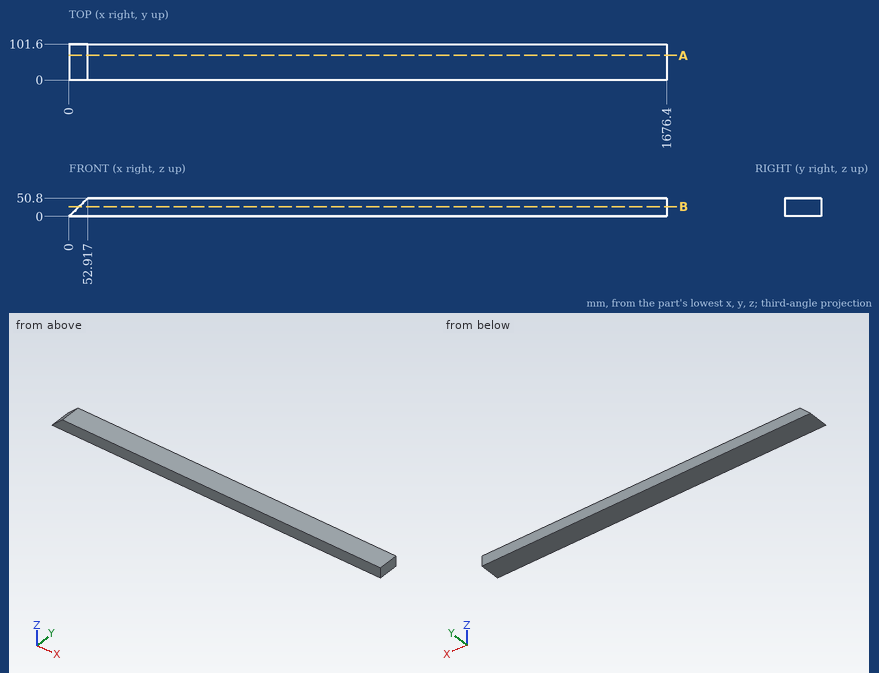
Input: dimensioned drawing with shaded views. Units: mm. Origin: part minimum x, y, z. Coordinates: 2 decimals unless noted, no trailing zeros. Write each loop counter-clockwise with the first axis right and the second up, starting at its lowest first coordinate (ties: lowest second). Pieces come first, ordered by that corner, then holes. Notation, with made-up numbers: M 28,12.25 L 36,12.25 A15 cw 36,34.25 Z; hole C 48.25,-10 d4. An arc over 180 degrees is marked long. Use one line per item in the form item = value.
Q1. Section A-A (y = 70). Return loops of the section in (x, z).
Answer below:
outline = M 0,0 L 1676.4,0 L 1676.4,50.8 L 52.92,50.8 Z
Q2. Section B-B (z = 27). Return loops of the section in (x, y) (1 decimal).
Answer below:
outline = M 28.1,0 L 1676.4,0 L 1676.4,101.6 L 28.1,101.6 Z
Q3. First-contact query: pin 1 (3 mm diameter, centred on y = 29.5, z = 14, fed in from -X). Flat tip, straight axial feed; report the tip coordinate or a pass-through.
Answer below:
pin_1 = 13.02
Q4. Material intervals for probe 1 along X at (y, z) = (13.5, 33.5) (1 decimal); probe 2 along X at (y, z) = (11, 36), sorted ascending. Write a range as from..to.
Answer below:
probe_1 = 34.9..1676.4
probe_2 = 37.5..1676.4
